```python
from build123d import *

# Parameters (mm, degrees)
CYLINDER004_R     = 5
CYLINDER004_DEPTH = 25.6
CYLINDER002_R     = 15
CYLINDER002_DEPTH = 2.8
CYLINDER001_R     = 15
CYLINDER001_DEPTH = 4.5
CYLINDER_R        = 18
CYLINDER_DEPTH    = 10.65
CYLINDER003_R     = 8
CYLINDER003_DEPTH = 13.6
FILLET_R          = 1
FILLET001_R       = 1


with BuildPart() as cylinder004:
    # Cylinder004 → Cylinder004 (new body)
    with BuildSketch(Plane.XY.offset(-1)):
        Circle(CYLINDER004_R)
    extrude(amount=CYLINDER004_DEPTH)


with BuildPart() as cylinder002:
    # Cylinder002 → Cylinder002 (new body)
    with BuildSketch(Plane.XY.offset(-0.5)):
        Circle(CYLINDER002_R)
    extrude(amount=CYLINDER002_DEPTH)


with BuildPart() as cylinder001:
    # Cylinder001 → Cylinder001 (new body)
    with BuildSketch(Plane.XY.offset(6.5)):
        Circle(CYLINDER001_R)
    extrude(amount=CYLINDER001_DEPTH)


with BuildPart() as cut001:
    # Cylinder → Cylinder (new body)
    with BuildSketch(Plane.XY):
        Circle(CYLINDER_R)
    extrude(amount=CYLINDER_DEPTH)

    # Cut: cut Cylinder001
    add(cylinder001.part, mode=Mode.SUBTRACT)

    # Cut001: cut Cylinder002
    add(cylinder002.part, mode=Mode.SUBTRACT)


with BuildPart() as body:
    # Cylinder003 → Cylinder003 (new body)
    with BuildSketch(Plane.XY.offset(2)):
        Circle(CYLINDER003_R)
    extrude(amount=CYLINDER003_DEPTH)

    # Fusion: union Cut001
    add(cut001.part)

    # Cut002: cut Cylinder004
    add(cylinder004.part, mode=Mode.SUBTRACT)

    # Fillet
    fillet_edges = [body.edges().sort_by_distance(p)[0] for p in [
        (-18, 0, 10.65),
    ]]
    fillet(fillet_edges, radius=FILLET_R)

    # Fillet001
    fillet001_edges = [body.edges().sort_by_distance(p)[0] for p in [
        (-18, 0, 0),
    ]]
    fillet(fillet001_edges, radius=FILLET001_R)


solid = body.part
```
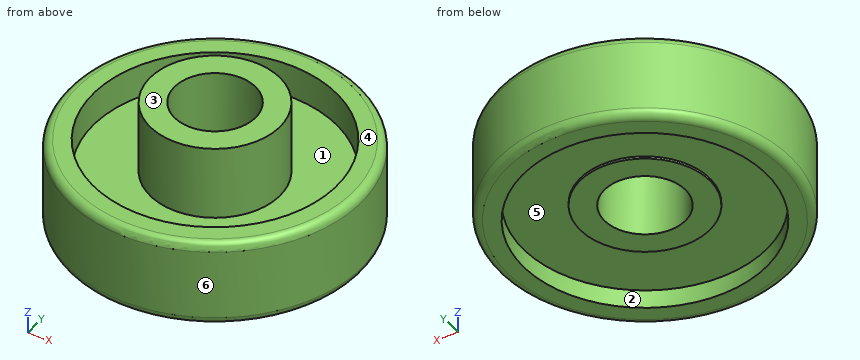
Input: part model. Units: mm. Frame: model coordinates. Face numbers are marked on the shaded views. A direction names the side the tool comes from. Round coordinates to 2 decimals unless told otherwise and drop trailing zeros. Loops run counter-clockwise (first coordinate to the right, second up) from the corner with the lowest first, then second, coordinate; pieces in that order, holes last.
1) Pin query (flat end, axial travel): pin 1 (5 mm diameter, centred on y = 4, z = 7, fed in from +X); pin 2 (6 mm diameter, centred on y = 9.5, z = 13, fed in from -X); pin 3 (16 mm diameter, centred on x = 0, y = 0, fed in from -Z). Return the tip coordinate at first contact, or that it passes through.
Ans:
pin 1: stops at x = 17.94
pin 2: stops at x = -15.76
pin 3: stops at z = 2
2) Section query D-D on z = 4. Return the cut outline in (x, y).
Ans:
outline: circle Ø36 at (0, 0); hole circle Ø10 at (0, 0)
3) Set-up query: the marked faces 1, 2 and 3. Return all of +Z, -Z, +X, -X, +Y, -Y with unobstructed straight access to the full face (end or side cutting, diameter ignored); none if empty.
Ans:
face 1: +Z
face 2: -Z
face 3: +Z, +X, -X, +Y, -Y
4) Section query A-A on z = 7. Return the cut outline in (x, y).
Ans:
outline: circle Ø36 at (0, 0); circle Ø16 at (0, 0); hole circle Ø30 at (0, 0); hole circle Ø10 at (0, 0)
5) Material intervals for line 1 (Y direction, x = 0, z = 7); line 2 (X direction, y = 4.5, z = 9.75); line 3 (Y direction, x = 0, z = 11.25), sorted ascending.
Ans:
line 1: y = -18 to -15, -8 to -5, 5 to 8, 15 to 18
line 2: x = -17.42 to -14.31, -6.61 to -2.18, 2.18 to 6.61, 14.31 to 17.42
line 3: y = -8 to -5, 5 to 8
6) Pull-direction query (Y, two-part tool) for the marked faces 4, 5 and 6; classes: released by +Y, released by -Y, zero draft, split by the parting line, or undercut.
Ans:
face 4: zero draft
face 5: undercut
face 6: split by the parting line
7) Section query B-B on y = 0. Return the cut outline in (x, z).
Ans:
outline: (-18, 1) arc R1 ccw to (-17, 0) - (-15, 0) - (-15, 2.3) - (-8, 2.3) - (-8, 2) - (-5, 2) - (-5, 15.6) - (-8, 15.6) - (-8, 6.5) - (-15, 6.5) - (-15, 10.65) - (-17, 10.65) arc R1 ccw to (-18, 9.65) - close; (5, 2) - (8, 2) - (8, 2.3) - (15, 2.3) - (15, 0) - (17, 0) arc R1 ccw to (18, 1) - (18, 9.65) arc R1 ccw to (17, 10.65) - (15, 10.65) - (15, 6.5) - (8, 6.5) - (8, 15.6) - (5, 15.6) - close
